from build123d import *

# Parameters (mm, degrees)
SKETCH1_R               = 34.5
BOSS_EXTRUDE1_DEPTH     = 4
CUT_EXTRUDE1_DEPTH      = 1
CUT_EXTRUDE1_DEPTH_BACK = 5
SKETCH6_R               = 20.912013364
BOSS_EXTRUDE2_DEPTH     = 5
CUT_EXTRUDE3_DEPTH      = 6
SKETCH7_R               = 3.5
CUT_EXTRUDE4_DEPTH      = 1
CUT_EXTRUDE4_DEPTH_BACK = 10
CUT_EXTRUDE5_DEPTH      = 2
SKETCH9_W               = 2
SKETCH9_H               = 3
CUT_EXTRUDE6_DEPTH      = 10


with BuildPart() as part:
    # Sketch1 → Boss-Extrude1 (new body)
    with BuildSketch(Plane(origin=(0, 0, 0), x_dir=(1, 0, 0), z_dir=(0, 1, 0))):
        Circle(SKETCH1_R)
    extrude(amount=BOSS_EXTRUDE1_DEPTH)

    # Sketch2 → Cut-Extrude1 (cut, two sides)
    with BuildSketch(Plane(origin=(0, 4, 0), x_dir=(1, 0, 0), z_dir=(0, 1, 0))) as cut_extrude1_sk:
        with BuildLine():
            ThreePointArc((18.645465696, -24.765835519), (30.69642547, -4.327755005), (24.765835519, 18.645465696))
            ThreePointArc((24.765835519, 18.645465696), (19.864559575, 19.336475193), (19.173550079, 14.435199249))
            ThreePointArc((19.173550079, 14.435199249), (23.764974557, -3.350520004), (14.435199249, -19.173550079))
            ThreePointArc((14.435199249, -19.173550079), (13.744189753, -24.074826023), (18.645465696, -24.765835519))
        make_face()
        with BuildLine():
            ThreePointArc((-14.435199249, 19.173550079), (-23.764974557, 3.350520004), (-19.173550079, -14.435199249))
            ThreePointArc((-19.173550079, -14.435199249), (-19.864559575, -19.336475193), (-24.765835519, -18.645465696))
            ThreePointArc((-24.765835519, -18.645465696), (-30.69642547, 4.327755005), (-18.645465696, 24.765835519))
            ThreePointArc((-18.645465696, 24.765835519), (-13.744189753, 24.074826023), (-14.435199249, 19.173550079))
        make_face()
    extrude(amount=CUT_EXTRUDE1_DEPTH, mode=Mode.SUBTRACT)
    extrude(cut_extrude1_sk.sketch, amount=-CUT_EXTRUDE1_DEPTH_BACK, mode=Mode.SUBTRACT)

    # Sketch6 → Boss-Extrude2 (add)
    with BuildSketch(Plane(origin=(0, 4, 0), x_dir=(1, 0, 0), z_dir=(0, 1, 0))):
        Circle(SKETCH6_R)
    extrude(amount=BOSS_EXTRUDE2_DEPTH)

    # Sketch5 → Cut-Extrude3 (cut)
    with BuildSketch(Plane(origin=(0, 9, 0), x_dir=(1, 0, 0), z_dir=(0, 1, 0))):
        with BuildLine():
            Line((-9, 0), (-9, -17))
            Line((-9, -17), (9, -17))
            Line((9, -17), (9, 0))
            ThreePointArc((9, 0), (0, 9), (-9, 0))
        make_face()
    extrude(amount=-CUT_EXTRUDE3_DEPTH, mode=Mode.SUBTRACT)

    # Sketch7 → Cut-Extrude4 (cut, two sides)
    with BuildSketch(Plane(origin=(0, 9, 0), x_dir=(1, 0, 0), z_dir=(0, 1, 0))) as cut_extrude4_sk:
        Circle(SKETCH7_R)
    extrude(amount=CUT_EXTRUDE4_DEPTH, mode=Mode.SUBTRACT)
    extrude(cut_extrude4_sk.sketch, amount=-CUT_EXTRUDE4_DEPTH_BACK, mode=Mode.SUBTRACT)

    # Sketch8 → Cut-Extrude5 (cut)
    with BuildSketch(Plane(origin=(0, 3, 0), x_dir=(1, 0, 0), z_dir=(0, 1, 0))):
        with BuildLine():
            Line((7.123903424, -5.5), (-7.123903424, -5.5))
            ThreePointArc((-7.123903424, -5.5), (-9, 0), (-7.123903424, 5.5))
            Line((-7.123903424, 5.5), (7.123903424, 5.5))
            ThreePointArc((7.123903424, 5.5), (9, 0), (7.123903424, -5.5))
        make_face()
    extrude(amount=-CUT_EXTRUDE5_DEPTH, mode=Mode.SUBTRACT)

    # Sketch9 → Cut-Extrude6 (cut, through all)
    with BuildSketch(Plane(origin=(0, 9, 0), x_dir=(1, 0, 0), z_dir=(0, 1, 0))):
        with Locations((7.763148871, 0.138067302)):
            Rectangle(SKETCH9_W, SKETCH9_H)
    extrude(amount=-CUT_EXTRUDE6_DEPTH, mode=Mode.SUBTRACT)


solid = part.part
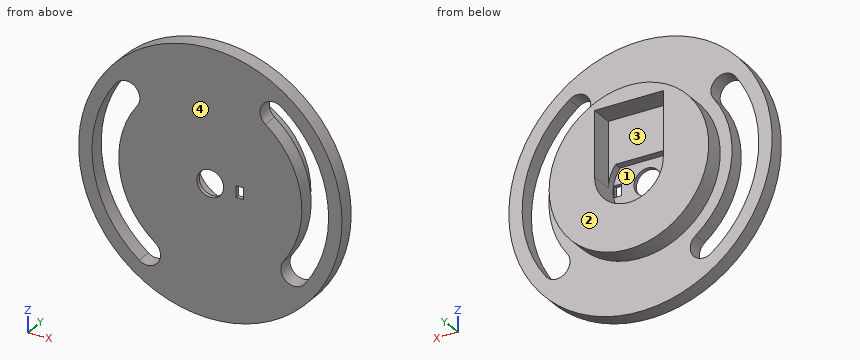
Model file for the job. Use its own axes, mm. Face numbers are marked on the shaded views. A direction names the side the tool comes from. Give positions to 0.01 mm unless a question says otherwise; leave off trailing zeros. Order: outer loops, then holes, each group sorted by start corner. A loop starts at its lowest first (then second) coordinate and runs counter-clockwise, first axis right, second up. Notation, with made-up numbers: (-21.5, 83) - (-8.5, 83) arc R10 cw to (-8.5, 88) - close; hole circle Ø9 at (64, 52.25). An arc over 180 degrees is marked (long way). Return JSON: item names as keys, results as strings.
1) Probe line 1 (X direction, y = 0.6, z = 0); line 2 (Z direction, x = 0, y = 0.4); line 3 (X direction, y = 1.75, z = 4.5). List the from-to ranges inside material, lowest first. Write a range as from..to.
Geometry says:
{"line 1": "-34.5..-31, -24..-3.5, 3.5..6.76, 8.76..24, 31..34.5", "line 2": "-34.5..-3.5, 3.5..34.5", "line 3": "-34.21..-30.67, -23.57..-7.79, 7.79..23.57, 30.67..34.21"}
2) Flat gauge pins, fed straight in: P1, Ø2, axis at y = 3, z = 18.5, coming from the +X side; P2, Ø1.8, axis at x = 2, z = -6.5, coming from the +Y side; P3, Ø4, axis at x = -26, z = 10.5, coming from the +Y side; P4, Ø4, axis at y = 3.5, z = -10, coming from the +X side. Where does each tip first touch, or does it go through?
Geometry says:
{"P1": "x = 29.73", "P2": "y = 3", "P3": "through", "P4": "x = 33.56"}
3) 3-axis set-ups, long thin cutter, end or side, ignore diameter. For the marked faces 1 and 2: which of +Z, -Z, +X, -X, +Y, -Y reach the whole face in a straight line?
Geometry says:
{"face 1": "+Y", "face 2": "+Z, -Z, +X, -X, +Y"}
4) Cut at B-B, the plane y = 2. Give the cut face in (x, z), plus the area to 3 significant figures.
Geometry says:
{"outline": "circle Ø69 at (0, 0); hole (-24.77, 18.65) arc R31 ccw to (-18.65, -24.77) arc R3.5 ccw to (-14.44, -19.17) arc R24 cw to (-19.17, 14.44) arc R3.5 ccw to start; hole (-7.12, -5.5) - (7.12, -5.5) arc R9 ccw to (7.12, 5.5) - (-7.12, 5.5) arc R9 ccw to start; hole (14.44, 19.17) arc R24 cw to (19.17, -14.44) arc R3.5 ccw to (24.77, -18.65) arc R31 ccw to (18.65, 24.77) arc R3.5 ccw to start", "area": "2,870 mm²"}
5) Cut at C-C, the plane z = -23.5. Give the cut face in (x, y).
Geometry says:
{"outline": "(-25.26, 0) - (-20.22, 0) - (-20.22, 4) - (-25.26, 4) - close; (-13.39, 0) - (25.26, 0) - (25.26, 4) - (-13.39, 4) - close"}
6) Pull direction X, two halves, no side cores. Call the marked faces 3 and 4: pulls with the +X half, pulls with the -X half, needs draft (parallel to the pull), parting line crosses it, or undercut.
Geometry says:
{"face 3": "undercut", "face 4": "needs draft"}
7) Cut at D-D, the plane x = 22.5. Give the cut face in (y, z), plus the area to 3 significant figures.
Geometry says:
{"outline": "(0, -26.15) - (4, -26.15) - (4, -20) - (0, -20) - close; (0, -8.35) - (4, -8.35) - (4, 8.35) - (0, 8.35) - close; (0, 21.32) - (4, 21.32) - (4, 26.15) - (0, 26.15) - close", "area": "111 mm²"}
8) Cut at A-A, the plane x = 0. Give the cut face in (y, z), plus the area to 3 significant figures.
Geometry says:
{"outline": "(0, -34.5) - (4, -34.5) - (4, -20.91) - (9, -20.91) - (9, -9) - (3, -9) - (3, -5.5) - (1, -5.5) - (1, -3.5) - (0, -3.5) - close; (0, 3.5) - (1, 3.5) - (1, 5.5) - (3, 5.5) - (3, 17) - (9, 17) - (9, 20.91) - (4, 20.91) - (4, 34.5) - (0, 34.5) - close", "area": "300 mm²"}
